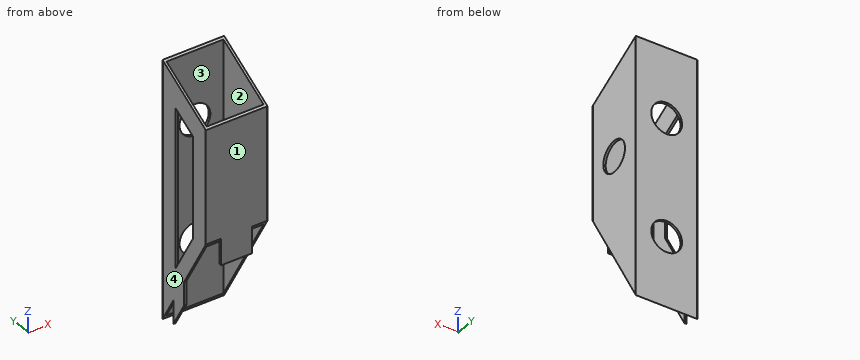
from build123d import *

# Parameters (mm, degrees)
SKETCH1_W           = 37
SKETCH1_H           = 37
BOSS_EXTRUDE1_DEPTH = 165.35
CUT_EXTRUDE1_DEPTH  = 50
BOSS_EXTRUDE2_START = -10
BOSS_EXTRUDE2_DEPTH = 20
BOSS_EXTRUDE3_DEPTH = 1.5
CUT_EXTRUDE2_DEPTH  = 10
SKETCH6_R           = 10
CUT_EXTRUDE3_DEPTH  = 10
SKETCH7_R           = 10
CUT_EXTRUDE4_DEPTH  = 10


with BuildPart() as part:
    # Sketch1 → Boss-Extrude1 (new body)
    with BuildSketch(Plane.XY):
        with BuildLine():
            Line((0.305025041, 0), (39.694974959, 0))
            ThreePointArc((39.694974959, 0), (39.910660234, 0.089339766), (40, 0.305025041))
            Line((40, 0.305025041), (40, 39.694974959))
            ThreePointArc((40, 39.694974959), (39.910660234, 39.910660234), (39.694974959, 40))
            Line((39.694974959, 40), (0.305025041, 40))
            ThreePointArc((0.305025041, 40), (0.089339766, 39.910660234), (0, 39.694974959))
            Line((0, 39.694974959), (0, 0.305025041))
            ThreePointArc((0, 0.305025041), (0.089339766, 0.089339766), (0.305025041, 0))
        make_face()
        with Locations((20, 20)):
            Rectangle(SKETCH1_W, SKETCH1_H, mode=Mode.SUBTRACT)
    extrude(amount=BOSS_EXTRUDE1_DEPTH)

    # Sketch2 → Cut-Extrude1 (cut)
    with BuildSketch(Plane(origin=(40, 0, 0), x_dir=(0, 0, -1), z_dir=(1, 0, 0))):
        Polygon((0, 40), (-69.282032303, 0), (0, 0), align=None)
        Polygon((-165.35, 40), (-142.255989232, 0), (-165.35, 0), align=None)
    extrude(amount=-CUT_EXTRUDE1_DEPTH, mode=Mode.SUBTRACT)

    # Sketch3 → Boss-Extrude2 (add)
    with BuildSketch(Plane.ZY.offset(BOSS_EXTRUDE2_START)):
        Polygon((69.282032303, 0), (52.282032303, 0), (52.282032303, 1.5), (66.683956091, 1.5), align=None)
    extrude(amount=-BOSS_EXTRUDE2_DEPTH)

    # Sketch4 → Boss-Extrude3 (add)
    with BuildSketch(Plane.ZY):
        Polygon((2.320508076, 30), (19.641016151, 20), (34.641016151, 20), (17.320508076, 30), align=None)
    extrude(amount=-BOSS_EXTRUDE3_DEPTH)

    # Sketch5 → Cut-Extrude2 (cut)
    with BuildSketch(Plane(origin=(0, 0, 0), x_dir=(0, 0, -1), z_dir=(1, 0, 0))):
        Polygon((-38.784609691, 28), (-66.497422612, 12), (-131.863684387, 12), (-141.101288694, 28), align=None)
    extrude(amount=CUT_EXTRUDE2_DEPTH, mode=Mode.SUBTRACT)

    # Sketch6 → Cut-Extrude3 (cut)
    with BuildSketch(Plane(origin=(0, 40, 0), x_dir=(1, 0, 0), z_dir=(0, 1, 0))):
        with Locations(Location((20, -120.35, 0), (0, 0, 180))):
            Circle(SKETCH6_R)
        with Locations(Location((20, -45, 0), (0, 0, 180))):
            Circle(SKETCH6_R)
    extrude(amount=-CUT_EXTRUDE3_DEPTH, mode=Mode.SUBTRACT)

    # Sketch7 → Cut-Extrude4 (cut)
    with BuildSketch(Plane.ZY.offset(-38.5)):
        with Locations((99.35, 20)):
            Circle(SKETCH7_R)
    extrude(amount=-CUT_EXTRUDE4_DEPTH, mode=Mode.SUBTRACT)


solid = part.part
CAD build for the part. Positions are in the model's coordinates, mm. Face numbers are marked on the shaded views. Coordinates: 2 decimals unless noted, no trailing zeros. Write each loop counter-clockwise with the first axis right and the second up, starting at its lowest first coordinate (ties: lowest second). Pieces come first, ordered by that corner, then holes. Notation, with made-up numbers: M 45.25,47.5 L 87.25,47.5 A25 ccw 87.25,85.5 Z; hole C 86.5,82.5 d9. An arc over 180 degrees is marked long. Return JSON: item names as keys, results as strings.
Item 1: Slice it at A-A, the plane x = 20. Write the cut outline in (y, z).
Findings below:
{"outline": "M 0,52.28 L 1.5,52.28 L 1.5,143.12 L 0,142.26 Z; M 38.5,2.6 L 40,0 L 40,35 L 38.5,35 Z; M 38.5,55 L 40,55 L 40,110.35 L 38.5,110.35 Z; M 38.5,130.35 L 40,130.35 L 40,165.35 L 38.5,164.48 Z"}
Item 2: Slice it at C-C, the plane y = 22.5. Write the cut outline in (x, z).
Findings below:
{"outline": "M 0,15.31 L 1.5,15.31 L 1.5,48.31 L 0,48.31 Z; M 0,137.93 L 1.5,137.93 L 1.5,155.25 L 0,155.25 Z; M 38.5,30.31 L 40,30.31 L 40,89.67 L 38.5,89.67 Z; M 38.5,109.03 L 40,109.03 L 40,155.25 L 38.5,155.25 Z"}
Item 3: Slice it at D-D, the plane y = 31.5. Write the cut outline in (x, z), and give its area (3 significant figures).
Findings below:
{"outline": "M 0,14.72 L 1.5,14.72 L 1.5,160.44 L 0,160.44 Z; M 38.5,14.72 L 40,14.72 L 40,160.44 L 38.5,160.44 Z", "area": "437 mm2"}
Item 4: Two-plate mould, pull along Y, no slides. Class the marked faces 1, 2, 3 and 4: +Y half, -Y half, draft (parallel to the pull), parting line (faces both ways), or undercut.
Findings below:
{"face 1": "-Y half", "face 2": "undercut", "face 3": "undercut", "face 4": "draft"}
Item 5: Slice it at B-B, the plane z = 120.35. Write the cut outline in (x, y), and give its area (3 significant figures).
Findings below:
{"outline": "M 0,0.31 A0.31 ccw 0.31,0 L 39.69,0 A0.31 ccw 40,0.31 L 40,39.69 A0.31 ccw 39.69,40 L 30,40 L 30,38.5 L 38.5,38.5 L 38.5,1.5 L 1.5,1.5 L 1.5,12 L 0,12 Z; M 0,28 L 1.5,28 L 1.5,38.5 L 10,38.5 L 10,40 L 0.31,40 A0.31 ccw 0,39.69 Z", "area": "177 mm2"}
Item 6: Drop flat-ended pins along their axis: pin 1 Ø0.8 at (x, y) = (22, 1) entering from -Z; pin 2 Ø6 at (y, z) = (14.5, 99.5) entering from +X; pin 3 Ø1.2 at (x, z) = (1, 26) entering from -Y. Give the stop position or say it passes through.
Findings below:
{"pin 1": "stops at z = 52.28", "pin 2": "stops at x = 1.5", "pin 3": "stops at y = 20"}
Item 7: Probe line 1 (X direction, y = 36, z = 80.5); line 2 (Y direction, x = 39.7, z = 99.35). List the from-to ranges inside material, lowest first. Write a range as from..to.
Findings below:
{"line 1": "x = 0..1.5, 38.5..40", "line 2": "y = 0..10, 30..40"}
